Source: CAD feature listing. Evaluate the final solid. Frame: model axes, mm. A direction names the side the tool comes from. Give positions to 0.01 mm unless a question says otherwise; leave off trailing zeros. Write each loop counter-clockwise with the first axis right and the second up, starting at its lowest first coordinate (ties: lowest second). Pieces come first, ordered by that corner, then holes. Notation, with made-up numbers: (86.25, 75.25) - (106.25, 75.25) arc R24 ccw to (106.25, 99.25) - close; hole circle Ø10 at (33, 53). An arc over 180 degrees is marked (long way). Answer as a JSON object with one key per item and string values. Group by question number.
from build123d import *

# Parameters (mm, degrees)
SKETCH3_W               = 70
SKETCH3_H               = 60
BOSS_EXTRUDE1_DEPTH     = 20
BOSS_EXTRUDE2_DEPTH     = 20
SKETCH5_R               = 0.75
CUT_EXTRUDE1_DEPTH      = 21
SKETCH7_R               = 0.75
CUT_EXTRUDE2_DEPTH      = 21
LPATTERN2_COUNT         = 3
LPATTERN2_PITCH         = 2
LPATTERN3_COUNT         = 3
LPATTERN3_PITCH         = 2
SKETCH8_W               = 250
SKETCH8_H               = 200
BOSS_EXTRUDE3_DEPTH     = 20
SKETCH9_W               = 230
SKETCH9_H               = 180
CUT_EXTRUDE3_DEPTH      = 19
SKETCH10_W              = 40
SKETCH10_H              = 40
BOSS_EXTRUDE4_DEPTH     = 30
SKETCH11_W              = 34
SKETCH11_H              = 34
CUT_EXTRUDE4_DEPTH      = 28.5
SKETCH19_W              = 5
SKETCH19_H              = 5
BOSS_EXTRUDE5_DEPTH     = 10
MIRROR2_COPY_1_SKETCH_W = 5
MIRROR2_COPY_1_SKETCH_H = 5
MIRROR2_COPY_1_DEPTH    = 10
SKETCH23_W              = 3
SKETCH23_H              = 3
BOSS_EXTRUDE6_DEPTH     = 28.5
MIRROR4_COPY_1_SKETCH_W = 3
MIRROR4_COPY_1_SKETCH_H = 3
MIRROR4_COPY_1_DEPTH    = 28.5
SKETCH27_R              = 3
CUT_EXTRUDE5_DEPTH      = 146
SKETCH28_R              = 2.5
CUT_EXTRUDE6_DEPTH      = 4
SKETCH29_R              = 0.225
CUT_EXTRUDE7_DEPTH      = 77
SKETCH30_R              = 0.225
CUT_EXTRUDE8_DEPTH      = 77
FILLET1_R               = 5
FILLET2_R               = 5


with BuildPart() as part:
    # Sketch3 → Boss-Extrude1 (new body)
    with BuildSketch(Plane.XY):
        with Locations((35, 30)):
            Rectangle(SKETCH3_W, SKETCH3_H)
    extrude(amount=BOSS_EXTRUDE1_DEPTH)

    # Sketch4 → Boss-Extrude2 (add)
    with BuildSketch(Plane.XY):
        with BuildLine():
            Line((0, 60), (0, 0))
            ThreePointArc((0, 0), (-30, 30), (0, 60))
        make_face()
        with BuildLine():
            Line((70, 60), (70, 0))
            ThreePointArc((70, 0), (100, 30), (70, 60))
        make_face()
    extrude(amount=BOSS_EXTRUDE2_DEPTH)

    # Sketch5 → Cut-Extrude1 (cut, through all)
    with BuildSketch(Plane.XY):
        with Locations((20.25, 30)):
            Circle(SKETCH5_R)
    cut_extrude1 = extrude(amount=CUT_EXTRUDE1_DEPTH, mode=Mode.SUBTRACT)

    # Sketch7 → Cut-Extrude2 (cut, through all)
    with BuildSketch(Plane.XY.offset(20)):
        with Locations((49.75, 30)):
            Circle(SKETCH7_R)
    cut_extrude2 = extrude(amount=-CUT_EXTRUDE2_DEPTH, mode=Mode.SUBTRACT)

    # LPattern2: Cut-Extrude1 ×3
    with Locations(*[(i * LPATTERN2_PITCH, 0, 0) for i in range(1, LPATTERN2_COUNT)]):
        add(cut_extrude1, mode=Mode.SUBTRACT)

    # LPattern3: Cut-Extrude2 ×3
    with Locations(*[(-i * LPATTERN3_PITCH, 0, 0) for i in range(1, LPATTERN3_COUNT)]):
        add(cut_extrude2, mode=Mode.SUBTRACT)

    # Sketch8 → Boss-Extrude3 (add)
    with BuildSketch(Plane(origin=(0, 60, 0), x_dir=(1, 0, 0), z_dir=(0, 1, 0))):
        with Locations((35, -10)):
            Rectangle(SKETCH8_W, SKETCH8_H)
    extrude(amount=BOSS_EXTRUDE3_DEPTH)

    # Sketch9 → Cut-Extrude3 (cut)
    with BuildSketch(Plane(origin=(0, 80, 0), x_dir=(1, 0, 0), z_dir=(0, 1, 0))):
        with Locations((35, -10)):
            Rectangle(SKETCH9_W, SKETCH9_H)
    extrude(amount=-CUT_EXTRUDE3_DEPTH, mode=Mode.SUBTRACT)

    # Sketch10 → Boss-Extrude4 (add)
    with BuildSketch(Plane.XZ.offset(-60)):
        with Locations((35, 65)):
            Rectangle(SKETCH10_W, SKETCH10_H)
    extrude(amount=BOSS_EXTRUDE4_DEPTH)

    # Sketch11 → Cut-Extrude4 (cut)
    with BuildSketch(Plane.XZ.offset(-30)):
        with Locations((35, 65)):
            Rectangle(SKETCH11_W, SKETCH11_H)
    extrude(amount=-CUT_EXTRUDE4_DEPTH, mode=Mode.SUBTRACT)

    # Sketch19 → Boss-Extrude5 (add)
    with BuildSketch(Plane.XZ.offset(-58.5)):
        with Locations((25.055, 74.81)):
            Rectangle(SKETCH19_W, SKETCH19_H)
    boss_extrude5 = extrude(amount=BOSS_EXTRUDE5_DEPTH)

    # Sketch22 → 3.0mm Dowel Hole1 (revolve, cut)
    with BuildSketch(Plane(origin=(23.755, 48.5, 76.11), x_dir=(0, 0, -1), z_dir=(1, 0, 0))):
        Polygon((0, 0), (0, 10.457855792), (0.762, 10), (0.762, 0), align=None)
    f_3_0mm_dowel_hole1 = revolve(axis=Axis((23.755, 42.15, 76.11), (0, 1, 0)), mode=Mode.SUBTRACT)

    # Mirror1: Boss-Extrude5, 3.0mm Dowel Hole1 across plane
    add(boss_extrude5.mirror(Plane(origin=(35, 0, 0), x_dir=(0, 0, 1), z_dir=(1, 0, 0))))
    add(f_3_0mm_dowel_hole1.mirror(Plane(origin=(35, 0, 0), x_dir=(0, 0, 1), z_dir=(1, 0, 0))), mode=Mode.SUBTRACT)

    # Mirror2: Boss-Extrude5, 3.0mm Dowel Hole1 across plane
    add(boss_extrude5.mirror(Plane.XY.offset(65)))
    add(f_3_0mm_dowel_hole1.mirror(Plane.XY.offset(65)), mode=Mode.SUBTRACT)

    # Mirror2 copy 1 sketch → Mirror2 copy 1 (add)
    with BuildSketch(Plane(origin=(70, 58.5, 130), x_dir=(-1, 0, 0), z_dir=(0, -1, 0))):
        with Locations((25.055, 74.81)):
            Rectangle(MIRROR2_COPY_1_SKETCH_W, MIRROR2_COPY_1_SKETCH_H)
    extrude(amount=MIRROR2_COPY_1_DEPTH)

    # Mirror2 copy 2 sketch → Mirror2 copy 2 (revolve, cut)
    with BuildSketch(Plane(origin=(46.245, 48.5, 53.89), x_dir=(0, 0, 1), z_dir=(-1, 0, 0))):
        Polygon((0, 0), (0, 10.457855792), (0.762, 10), (0.762, 0), align=None)
    revolve(axis=Axis((46.245, 42.15, 53.89), (0, 1, 0)), mode=Mode.SUBTRACT)

    # Sketch23 → Boss-Extrude6 (add)
    with BuildSketch(Plane.XZ.offset(-58.5)):
        with Locations((19.5, 80.5)):
            Rectangle(SKETCH23_W, SKETCH23_H)
    boss_extrude6 = extrude(amount=BOSS_EXTRUDE6_DEPTH)

    # Mirror3: Boss-Extrude6 across plane
    add(boss_extrude6.mirror(Plane.XY.offset(65)))

    # Mirror4: Boss-Extrude6 across plane
    add(boss_extrude6.mirror(Plane(origin=(35, 0, 0), x_dir=(0, 0, 1), z_dir=(1, 0, 0))))

    # Mirror4 copy 1 sketch → Mirror4 copy 1 (add)
    with BuildSketch(Plane(origin=(70, 58.5, 130), x_dir=(-1, 0, 0), z_dir=(0, -1, 0))):
        with Locations((19.5, 80.5)):
            Rectangle(MIRROR4_COPY_1_SKETCH_W, MIRROR4_COPY_1_SKETCH_H)
    extrude(amount=MIRROR4_COPY_1_DEPTH)

    # Sketch26 → 3.0mm Dowel Hole2 (revolve, cut)
    with BuildSketch(Plane(origin=(18, 30, 82), x_dir=(0, 0, -1), z_dir=(1, 0, 0))):
        Polygon((0, 0), (0, 10.901290929), (1.5, 10), (1.5, 0), align=None)
    f_3_0mm_dowel_hole2 = revolve(axis=Axis((18, 23.65, 82), (0, 1, 0)), mode=Mode.SUBTRACT)

    # Mirror5: 3.0mm Dowel Hole2 across plane
    add(f_3_0mm_dowel_hole2.mirror(Plane.XY.offset(65)), mode=Mode.SUBTRACT)

    # Mirror6: 3.0mm Dowel Hole2 across plane
    add(f_3_0mm_dowel_hole2.mirror(Plane(origin=(35, 0, 0), x_dir=(0, 0, 1), z_dir=(1, 0, 0))), mode=Mode.SUBTRACT)

    # Mirror6 copy 1 sketch → Mirror6 copy 1 (revolve, cut)
    with BuildSketch(Plane(origin=(52, 30, 48), x_dir=(0, 0, 1), z_dir=(-1, 0, 0))):
        Polygon((0, 0), (0, 10.901290929), (1.5, 10), (1.5, 0), align=None)
    revolve(axis=Axis((52, 23.65, 48), (0, 1, 0)), mode=Mode.SUBTRACT)

    # Sketch27 → Cut-Extrude5 (cut, through all)
    with BuildSketch(Plane(origin=(55, 0, 0), x_dir=(0, 0, -1), z_dir=(1, 0, 0))):
        with Locations((-65, 40)):
            Circle(SKETCH27_R)
    extrude(amount=-CUT_EXTRUDE5_DEPTH, mode=Mode.SUBTRACT)

    # Sketch28 → Cut-Extrude6 (cut)
    with BuildSketch(Plane(origin=(0, 80, 0), x_dir=(1, 0, 0), z_dir=(0, 1, 0))):
        with Locations((-85, -10)):
            Circle(SKETCH28_R)
    cut_extrude6 = extrude(amount=-CUT_EXTRUDE6_DEPTH, mode=Mode.SUBTRACT)

    # Sketch29 → Cut-Extrude7 (cut, through all)
    with BuildSketch(Plane(origin=(0, 76, 0), x_dir=(1, 0, 0), z_dir=(0, 1, 0))):
        with Locations((-85, -8.3)):
            Circle(SKETCH29_R)
    cut_extrude7 = extrude(amount=-CUT_EXTRUDE7_DEPTH, mode=Mode.SUBTRACT)

    # Sketch30 → Cut-Extrude8 (cut, through all)
    with BuildSketch(Plane(origin=(0, 76, 0), x_dir=(1, 0, 0), z_dir=(0, 1, 0))):
        with Locations((-85, -11.7)):
            Circle(SKETCH30_R)
    cut_extrude8 = extrude(amount=-CUT_EXTRUDE8_DEPTH, mode=Mode.SUBTRACT)

    # Mirror7: Cut-Extrude6, Cut-Extrude7, Cut-Extrude8 across plane
    add(cut_extrude6.mirror(Plane.ZY.offset(-35)), mode=Mode.SUBTRACT)
    add(cut_extrude7.mirror(Plane.ZY.offset(-35)), mode=Mode.SUBTRACT)
    add(cut_extrude8.mirror(Plane.ZY.offset(-35)), mode=Mode.SUBTRACT)

    # Fillet1
    fillet1_edges = [part.edges().sort_by_distance(p)[0] for p in [
        (-90, 70, -90),
        (-90, 70, 110),
        (160, 70, 110),
        (160, 70, -90),
    ]]
    fillet(fillet1_edges, radius=FILLET1_R)

    # Fillet2
    fillet2_edges = [part.edges().sort_by_distance(p)[0] for p in [
        (15, 45, 85),
        (15, 45, 45),
        (55, 45, 45),
        (55, 45, 85),
    ]]
    fillet(fillet2_edges, radius=FILLET2_R)


solid = part.part
Q1. First-contact query: pin 1 Ø1.5 at (x, y) = (44, 52.5) entering from -Z; pin 2 Ø2.5 at (x, z) = (24.5, 54) entering from -Y; pin 3 Ø1.2 at (x, z) = (46.245, 76.11) entering from +Y. Flat tips, straight axial feed; report the tip coordinate or a pass-through.
Q2. Ray query, probe 1 along X at (y, z) = (56.75, 76.11) (3 decimals); probe 2 along X at (y, z) = (66.25, 11.7) (3 decimals); probe 3 along Z at (x, y) = (-85, 72) (3 decimals). Return the intervals inside material, ascending. Write a range as [from, to].
Q3. Section A-A on z = 3. Return the cut outline in (x, y), then the cut area to 3 significant figures.
Q4. Section C-C on y = 69.5. Return the cut outline in (x, z) (3 decimals), then the cut area to 3 significant figures.
Q5. Draft query along Z for faces 1 (the flat face through (36, 30, 0)), 2 (the flat face through (35, 30, 83)), 3 (the flat face through (35, 58.5, 65)), 4 (the flat face through (45, 48.5, 55)). Return one class per face: released by +Z, released by -Z, zero draft, split by the parting line, or undercut.
Q6. Reachability of faces 5 (the cylindrical face through (-89, 70, -88)), 6 (the flat face through (150, 71, 11)), 7 (the cylindrical face through (53, 45, 46)), 8 (the flat face through (45, 48.5, 75)) from +Z, -Z, +X, -X, +Y, -Y: full face, straight path, thin tool, end or side. Return the list, or none.
Q7. Section D-D on z = -71.5. Return the cut outline in (x, y), then the cut area to 3 significant figures.
Q8. Section B-B on x = -15. Return the cut outline in (y, z).
Taken from the geometry:
{
 "1": {"pin 1": "stops at z = 0", "pin 2": "stops at y = 48.5", "pin 3": "stops at y = 61"},
 "2": {"probe 1": "x = [15, 18], [22.555, 22.993], [24.517, 27.555], [42.445, 45.483], [47.007, 47.445], [52, 55]", "probe 2": "x = [-90, -85.225], [-84.775, -80], [150, 154.775], [155.225, 160]", "probe 3": "z = [-90, 8.075], [8.525, 11.475], [11.925, 110]"},
 "3": {"outline": "(-90, 60) - (0, 60) arc R30 ccw to (0, 0) - (70, 0) arc R30 ccw to (70, 60) - (160, 60) - (160, 80) - (150, 80) - (150, 61) - (-80, 61) - (-80, 80) - (-90, 80) - close; hole circle Ø1.5 at (20.25, 30); hole circle Ø1.5 at (22.25, 30); hole circle Ø1.5 at (24.25, 30); hole circle Ø1.5 at (45.75, 30); hole circle Ø1.5 at (47.75, 30); hole circle Ø1.5 at (49.75, 30)", "area": "7,650 mm²"},
 "4": {"outline": "(-90, -85) arc R5 ccw to (-85, -90) - (155, -90) arc R5 ccw to (160, -85) - (160, 105) arc R5 ccw to (155, 110) - (-85, 110) arc R5 ccw to (-90, 105) - close; hole circle Ø0.45 at (-85, 8.3); hole circle Ø0.45 at (-85, 11.7); hole (-80, -80) - (150, -80) - (150, 100) - (-80, 100) - close; hole circle Ø0.45 at (155, 8.3); hole circle Ø0.45 at (155, 11.7)", "area": "8,580 mm²"},
 "5": {"face 1": "released by -Z", "face 2": "zero draft", "face 3": "undercut", "face 4": "undercut"},
 "6": {"face 5": "-Z, -X, +Y, -Y", "face 6": "+Y", "face 7": "+X, -Y", "face 8": "-Y"},
 "7": {"outline": "(-90, 60) - (160, 60) - (160, 80) - (150, 80) - (150, 61) - (-80, 61) - (-80, 80) - (-90, 80) - close", "area": "630 mm²"},
 "8": {"outline": "(4.02, 0) - (55.98, 0) - (55.98, 20) - (4.02, 20) - close; (60, -90) - (80, -90) - (80, -80) - (61, -80) - (61, 100) - (80, 100) - (80, 110) - (60, 110) - close"}
}
